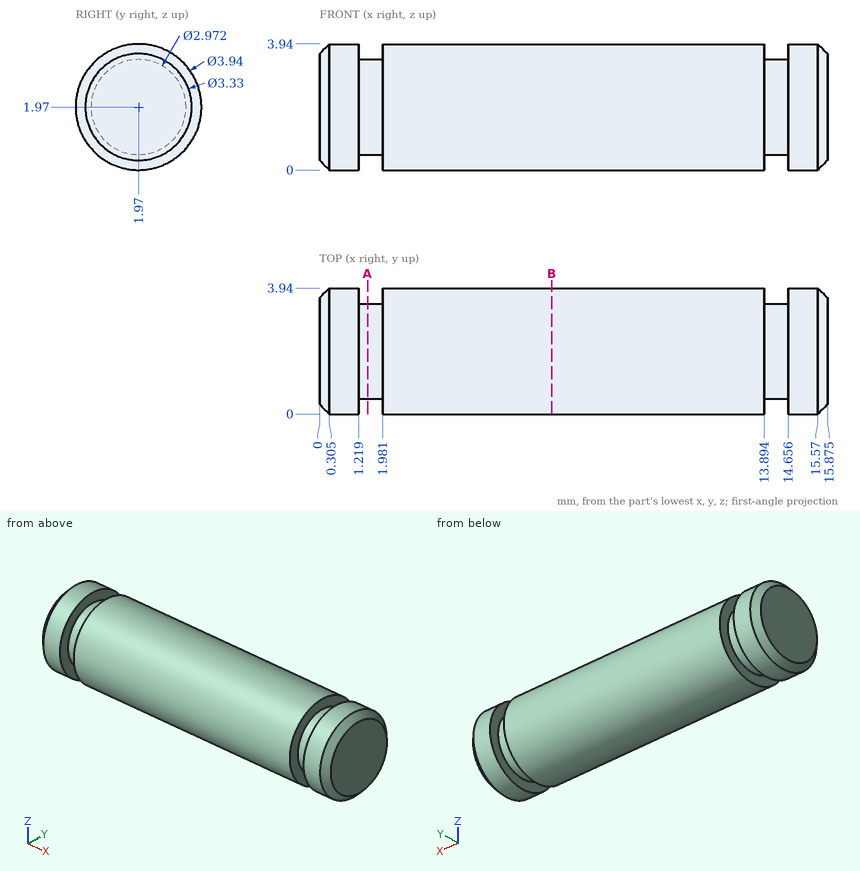
Check sheet for the drawn part. Datum: minimum x, y, z corner. Units: mm. Coordinates: 2 decimals unless noted, no trailing zeros. Loops run counter-clockwise (first coordinate to the right, second up) from the corner with the lowest first, then second, coordinate; pieces in that order, holes last. Notation, with made-up numbers: M -2,56 L 8,56 A31 ccw 8,95 Z; hole C 78.25,23.25 d4. An arc over 180 degrees is marked long. Answer as a JSON object with one key per item and string values.
1. Depth check by flat-ended pin: P1, Ø1.2, axis at y = 2, z = 1, coming from the -X side. Enter the tip coordinate at first touch or a pass-through.
Outcome:
{"P1": "x = 0"}
2. Sectioned sample at B-B on x = 7.25. Record the cut outline in (y, z), and give its area (3 significant figures).
Outcome:
{"outline": "C 1.97,1.97 d3.94", "area": "12.2 mm²"}
3. Sectioned sample at A-A on x = 1.5. Record the cut outline in (y, z) (1 decimal).
Outcome:
{"outline": "C 2,2 d3"}
4. Scan lines: L1, parallel to X at y = 1.15, z = 0.7 (1 decimal); L2, parallel to X at y = 0.65, z = 0.85 (1 decimal); L3, parallel to Z at x = 4, y = 1.9. Record each from-to range of solid material in increasing order. Write a range as from..to.
Outcome:
{"L1": "0..1.2, 2..13.9, 14.7..15.9", "L2": "0.1..1.2, 2..13.9, 14.7..15.8", "L3": "0..3.94"}
